Design review of the part built by this model. Coordinates are the model's own, in mm. Face numbers are marked on the shaded views. A direction names the side the tool comes from. Give positions to 0.01 mm unless a question says otherwise; leave off trailing zeros. Loops run counter-clockwise (first coordinate to the right, second up) from the corner with the lowest first, then second, coordinate; pieces in that order, holes last. Notation, with made-up numbers: M 74,-13.5 L 95,-13.5 A16 cw 95,17.5 Z; hole C 79,21 d8. An arc over 180 degrees is marked long. Use CSV: the item, a comma, the result in double quotes.
from build123d import *

# Parameters (mm, degrees)
SKETCH1_R           = 2.6035
BOSS_EXTRUDE1_DEPTH = 25.4


with BuildPart() as part:
    # Sketch1 → Boss-Extrude1 (new body)
    with BuildSketch(Plane(origin=(0, 0, 0), x_dir=(0, 0, -1), z_dir=(1, 0, 0))):
        with BuildLine():
            Line((6.333126718, -12.7), (9.550443118, -12.7))
            ThreePointArc((9.550443118, -12.7), (10.058366869, -12.192000006), (10.566443095, -12.699847501))
            ThreePointArc((10.566443095, -12.699847501), (12.082537762, -12.08250727), (12.699846982, -10.566399977))
            ThreePointArc((12.699846982, -10.566399977), (12.192000006, -10.058323491), (12.7, -9.5504))
            Line((12.7, -9.5504), (12.7, -6.3330836))
            ThreePointArc((12.7, -6.3330836), (12.192, -5.8250836), (12.7, -5.3170836))
            Line((12.7, -5.3170836), (12.7, -4.287469289))
            ThreePointArc((12.7, -4.287469289), (12.39275138, -3.545705502), (11.650987593, -3.238456882))
            Line((11.650987593, -3.238456882), (11.539212407, -3.238456882))
            ThreePointArc((11.539212407, -3.238456882), (10.79744862, -3.545705502), (10.4902, -4.287469289))
            Line((10.4902, -4.287469289), (10.4902, -6.402089023))
            ThreePointArc((10.4902, -6.402089023), (9.856505071, -7.351067942), (8.737131347, -7.129408934))
            Line((8.737131347, -7.129408934), (4.5085, -2.9104418))
            Line((4.5085, -2.9104418), (4.5085, 1.593185507))
            ThreePointArc((4.5085, 1.593185507), (4.750877967, 2.809883091), (5.441005833, 3.840816462))
            Line((5.441005833, 3.840816462), (8.737131347, 7.129408934))
            ThreePointArc((8.737131347, 7.129408934), (9.856505071, 7.351067942), (10.4902, 6.402089023))
            Line((10.4902, 6.402089023), (10.4902, 4.287469289))
            ThreePointArc((10.4902, 4.287469289), (10.79744862, 3.545705502), (11.539212407, 3.238456882))
            Line((11.539212407, 3.238456882), (11.650987593, 3.238456882))
            ThreePointArc((11.650987593, 3.238456882), (12.39275138, 3.545705502), (12.7, 4.287469289))
            Line((12.7, 4.287469289), (12.7, 5.3170836))
            ThreePointArc((12.7, 5.3170836), (12.192, 5.8250836), (12.7, 6.3330836))
            Line((12.7, 6.3330836), (12.7, 9.5504))
            ThreePointArc((12.7, 9.5504), (12.192000006, 10.058323491), (12.699846982, 10.566399977))
            ThreePointArc((12.699846982, 10.566399977), (12.082537762, 12.08250727), (10.566443095, 12.699847501))
            ThreePointArc((10.566443095, 12.699847501), (10.058366869, 12.192000006), (9.550443118, 12.7))
            Line((9.550443118, 12.7), (6.333126718, 12.7))
            ThreePointArc((6.333126718, 12.7), (5.825126718, 12.192), (5.317126718, 12.7))
            Line((5.317126718, 12.7), (4.287512407, 12.7))
            ThreePointArc((4.287512407, 12.7), (3.54574862, 12.39275138), (3.2385, 11.650987593))
            Line((3.2385, 11.650987593), (3.2385, 11.539212407))
            ThreePointArc((3.2385, 11.539212407), (3.54574862, 10.79744862), (4.287512407, 10.4902))
            Line((4.287512407, 10.4902), (6.476788598, 10.4902))
            ThreePointArc((6.476788598, 10.4902), (7.432222385, 9.85140422), (7.207036008, 8.724370562))
            Line((7.207036008, 8.724370562), (3.898272566, 5.423169045))
            ThreePointArc((3.898272566, 5.423169045), (2.869120213, 4.736787962), (1.655778399, 4.4958))
            Line((1.655778399, 4.4958), (-1.655778399, 4.4958))
            ThreePointArc((-1.655778399, 4.4958), (-2.869120213, 4.736787962), (-3.898272566, 5.423169045))
            Line((-3.898272566, 5.423169045), (-7.207036008, 8.724370562))
            ThreePointArc((-7.207036008, 8.724370562), (-7.432222385, 9.85140422), (-6.476788598, 10.4902))
            Line((-6.476788598, 10.4902), (-4.287512407, 10.4902))
            ThreePointArc((-4.287512407, 10.4902), (-3.54574862, 10.79744862), (-3.2385, 11.539212407))
            Line((-3.2385, 11.539212407), (-3.2385, 11.650987593))
            ThreePointArc((-3.2385, 11.650987593), (-3.54574862, 12.39275138), (-4.287512407, 12.7))
            Line((-4.287512407, 12.7), (-5.317126718, 12.7))
            ThreePointArc((-5.317126718, 12.7), (-5.825126718, 12.192), (-6.333126718, 12.7))
            Line((-6.333126718, 12.7), (-9.550443118, 12.7))
            ThreePointArc((-9.550443118, 12.7), (-10.058366869, 12.192000006), (-10.566443095, 12.699847501))
            ThreePointArc((-10.566443095, 12.699847501), (-12.082537762, 12.08250727), (-12.699846982, 10.566399977))
            ThreePointArc((-12.699846982, 10.566399977), (-12.192000006, 10.058323491), (-12.7, 9.5504))
            Line((-12.7, 9.5504), (-12.7, 6.3330836))
            ThreePointArc((-12.7, 6.3330836), (-12.192, 5.8250836), (-12.7, 5.3170836))
            Line((-12.7, 5.3170836), (-12.7, 4.287469289))
            ThreePointArc((-12.7, 4.287469289), (-12.39275138, 3.545705502), (-11.650987593, 3.238456882))
            Line((-11.650987593, 3.238456882), (-11.539212407, 3.238456882))
            ThreePointArc((-11.539212407, 3.238456882), (-10.79744862, 3.545705502), (-10.4902, 4.287469289))
            Line((-10.4902, 4.287469289), (-10.4902, 6.402089023))
            ThreePointArc((-10.4902, 6.402089023), (-9.856505071, 7.351067942), (-8.737131347, 7.129408934))
            Line((-8.737131347, 7.129408934), (-5.441005833, 3.840816462))
            ThreePointArc((-5.441005833, 3.840816462), (-4.750877967, 2.809883091), (-4.5085, 1.593185507))
            Line((-4.5085, 1.593185507), (-4.5085, -1.593185507))
            ThreePointArc((-4.5085, -1.593185507), (-4.750877967, -2.809883091), (-5.441005833, -3.840816462))
            Line((-5.441005833, -3.840816462), (-8.737131347, -7.129408934))
            ThreePointArc((-8.737131347, -7.129408934), (-9.856505071, -7.351067942), (-10.4902, -6.402089023))
            Line((-10.4902, -6.402089023), (-10.4902, -4.287469289))
            ThreePointArc((-10.4902, -4.287469289), (-10.79744862, -3.545705502), (-11.539212407, -3.238456882))
            Line((-11.539212407, -3.238456882), (-11.650987593, -3.238456882))
            ThreePointArc((-11.650987593, -3.238456882), (-12.39275138, -3.545705502), (-12.7, -4.287469289))
            Line((-12.7, -4.287469289), (-12.7, -5.3170836))
            ThreePointArc((-12.7, -5.3170836), (-12.192, -5.8250836), (-12.7, -6.3330836))
            Line((-12.7, -6.3330836), (-12.7, -9.5504))
            ThreePointArc((-12.7, -9.5504), (-12.192000006, -10.058323491), (-12.699846982, -10.566399977))
            ThreePointArc((-12.699846982, -10.566399977), (-12.082537762, -12.08250727), (-10.566443095, -12.699847501))
            ThreePointArc((-10.566443095, -12.699847501), (-10.058366869, -12.192000006), (-9.550443118, -12.7))
            Line((-9.550443118, -12.7), (-6.333126718, -12.7))
            ThreePointArc((-6.333126718, -12.7), (-5.825126718, -12.192), (-5.317126718, -12.7))
            Line((-5.317126718, -12.7), (-4.287512407, -12.7))
            ThreePointArc((-4.287512407, -12.7), (-3.54574862, -12.39275138), (-3.2385, -11.650987593))
            Line((-3.2385, -11.650987593), (-3.2385, -11.539212407))
            ThreePointArc((-3.2385, -11.539212407), (-3.54574862, -10.79744862), (-4.287512407, -10.4902))
            Line((-4.287512407, -10.4902), (-6.416408329, -10.4902))
            ThreePointArc((-6.416408329, -10.4902), (-7.41473083, -9.822813117), (-7.179650497, -8.645192506))
            Line((-7.179650497, -8.645192506), (-3.952270251, -5.423690499))
            ThreePointArc((-3.952270251, -5.423690499), (-2.922936451, -4.736929036), (-1.709253557, -4.4958))
            Line((-1.709253557, -4.4958), (1.709253557, -4.4958))
            ThreePointArc((1.709253557, -4.4958), (2.922936451, -4.736929036), (3.952270251, -5.423690499))
            Line((3.952270251, -5.423690499), (7.179650497, -8.645192506))
            ThreePointArc((7.179650497, -8.645192506), (7.41473083, -9.822813117), (6.416408329, -10.4902))
            Line((6.416408329, -10.4902), (4.287512407, -10.4902))
            ThreePointArc((4.287512407, -10.4902), (3.54574862, -10.79744862), (3.2385, -11.539212407))
            Line((3.2385, -11.539212407), (3.2385, -11.650987593))
            ThreePointArc((3.2385, -11.650987593), (3.54574862, -12.39275138), (4.287512407, -12.7))
            Line((4.287512407, -12.7), (5.317126718, -12.7))
            ThreePointArc((5.317126718, -12.7), (5.825126718, -12.192), (6.333126718, -12.7))
        make_face()
        Circle(SKETCH1_R, mode=Mode.SUBTRACT)
    extrude(amount=BOSS_EXTRUDE1_DEPTH)


solid = part.part
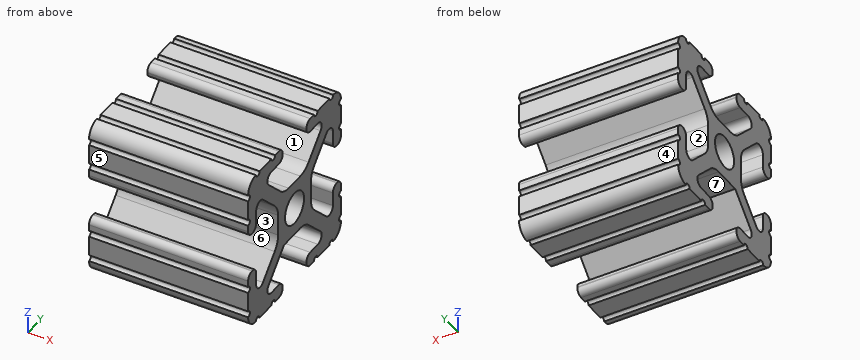
(1) Machinability: for the marked faces 1, 2, 3 and 4, which of the approach directions +Z, -Z, +X, -X, +Y, -Y give a long, thin tool a straight path to every point of the face, cutting with its end or side? Answer none if there is none.
A:
face 1,"+X, -X"
face 2,"+X, -X, +Y"
face 3,"+X, -X, -Y"
face 4,"+Z, -Z, +X, -X, +Y"
(2) We need section A-A on y = 0. State the section outline as (x, z) points, then the cut area to 3 significant figures.
A:
outline,"M 0,-4.51 L 25.4,-4.51 L 25.4,-2.6 L 0,-2.6 Z; M 0,2.6 L 25.4,2.6 L 25.4,4.51 L 0,4.51 Z"
area,"96.8 mm²"
(3) Wall thickness on line 1 along Y through (x, z) = (19.75, -6); line 2 along Y through (x, z) = (13.25, -7.25); line 3 along Y through (x, z) = (5.75, 0): over which ranges is each line inside the solid? List them lowest first. Write a range as [from, to].
A:
line 1,"[-12.22, -10.49], [-7.47, -4.4], [4.4, 7.52], [10.49, 12.22]"
line 2,"[-12.7, -10.1], [-8.72, -5.65], [5.65, 8.77], [10.14, 12.7]"
line 3,"[-4.5, -2.6], [2.6, 4.5]"
(4) We need section B-B on z = 0. State the section outline as (x, y) points.
A:
outline,"M 0,-4.5 L 25.4,-4.5 L 25.4,-2.6 L 0,-2.6 Z; M 0,2.6 L 25.4,2.6 L 25.4,4.5 L 0,4.5 Z"
(5) The part is to be moulded in two halves that separate along Z. For the marked faces 5, 6 and 7, say which applies: released by +Z, released by -Z, zero draft, split by the parting line, or undercut.
A:
face 5,"zero draft"
face 6,"undercut"
face 7,"released by -Z"
(6) Clearance check with flat-ended pins moving along their axes: P1, Ø2.5, axis at x = 14.5, y = -0.5, coming from the -Z side; P2, Ø1, axis at y = 4.5, z = -9.5, coming from the -X side; P3, Ø1, axis at x = 14.5, z = 0, coming from the -Y side; P4, Ø1, axis at x = 17, y = 0.5, coming from the +Z side. State where each tip first meets the part, or that it passes through.
A:
P1,"z = -4.51"
P2,"through"
P3,"y = -4.5"
P4,"z = 4.51"
